```python
from build123d import *

# Parameters (mm, degrees)
F0_W     = 3.5
F0_H     = 11
F1_DEPTH = 10
F2_R     = 3
F3_R     = 15.5
F4_DEPTH = 25
F3_W     = 3.5
F3_H     = 5
F5_DEPTH = 3
F6_R     = 2
F7_R     = 15.5
F8_DEPTH = 10


with BuildPart() as f1:
    # F0 (on Top) → F1 (new body)
    with BuildSketch(Plane.XY):
        with BuildLine():
            ThreePointArc((0, -19.5), (13.7885822331, -13.7885822331), (19.5, 0))
            ThreePointArc((19.5, 0), (13.7885822331, 13.7885822331), (0, 19.5))
            ThreePointArc((0, 19.5), (-19.5, 0), (0, -19.5))
        make_face()
        with BuildLine():
            ThreePointArc((0, 19.5), (13.7885822331, 13.7885822331), (19.5, 0))
            ThreePointArc((19.5, 0), (13.7885822331, -13.7885822331), (0, -19.5))
            Line((0, -19.5), (21.5, -19.5))
            Line((21.5, -19.5), (21.5, 19.5))
            Line((21.5, 19.5), (0, 19.5))
        make_face()
        Polygon((30.5, 16), (21.5, 19.5), (21.5, -19.5), (30.5, -16), (30.5, -5.5), (30.5, 5.5), align=None)
        with Locations((32.25, 0)):
            Rectangle(F0_W, F0_H)
    extrude(amount=F1_DEPTH)

    # F2
    f2_edges = [f1.edges().sort_by_distance(p)[0] for p in [
        (30.5, 16, 5),
        (21.5, 19.5, 5),
        (30.5, -16, 5),
        (21.5, -19.5, 5),
    ]]
    fillet(f2_edges, radius=F2_R)

    # F3 (on face) → F4 (cut)
    with BuildSketch(Plane.XY.offset(10)):
        Circle(F3_R)
        with BuildLine():
            Line((20.9371966075, 16.5), (10.3923048454, 16.5))
            ThreePointArc((10.3923048454, 16.5), (17.0719059347, 9.4233766643), (19.5, 0))
            ThreePointArc((19.5, 0), (17.0719059347, -9.4233766643), (10.3923048454, -16.5))
            Line((10.3923048454, -16.5), (20.9371966075, -16.5))
            Line((20.9371966075, -16.5), (27.5, -13.9477986807))
            Line((27.5, -13.9477986807), (27.5, -2.5))
            Line((27.5, -2.5), (27.5, 2.5))
            Line((27.5, 2.5), (27.5, 13.9477986807))
            Line((27.5, 13.9477986807), (20.9371966075, 16.5))
        make_face()
    extrude(amount=-F4_DEPTH, mode=Mode.SUBTRACT)

    # F3 (on face) → F5 (join)
    with BuildSketch(Plane.XY.offset(10)):
        with BuildLine():
            Line((20.9371966075, 24.5), (0, 24.5))
            ThreePointArc((0, 24.5), (-24.5, 0), (0, -24.5))
            Line((0, -24.5), (20.9371966075, -24.5))
            ThreePointArc((20.9371966075, -24.5), (22.4122730498, -24.3628334263), (23.8367666967, -23.9560373723))
            Line((23.8367666967, -23.9560373723), (30.3995700892, -21.403836053))
            ThreePointArc((30.3995700892, -21.403836053), (34.1028993902, -18.4646249606), (35.5, -13.9477986807))
            Line((35.5, -13.9477986807), (35.5, -10.5))
            Line((35.5, -10.5), (39, -10.5))
            Line((39, -10.5), (39, 10.5))
            Line((39, 10.5), (35.5, 10.5))
            Line((35.5, 10.5), (35.5, 13.9477986807))
            ThreePointArc((35.5, 13.9477986807), (34.1028993902, 18.4646249606), (30.3995700892, 21.403836053))
            Line((30.3995700892, 21.403836053), (23.8367666967, 23.9560373723))
            ThreePointArc((23.8367666967, 23.9560373723), (22.4122730498, 24.3628334263), (20.9371966075, 24.5))
        make_face()
        with BuildLine():
            ThreePointArc((0, -19.5), (-19.5, 0), (0, 19.5))
            Line((0, 19.5), (20.9371966075, 19.5))
            ThreePointArc((20.9371966075, 19.5), (21.4903502734, 19.4485625349), (22.024535391, 19.2960140146))
            Line((22.024535391, 19.2960140146), (28.5873387835, 16.7438126953))
            ThreePointArc((28.5873387835, 16.7438126953), (29.9760872713, 15.6416085357), (30.5, 13.9477986807))
            Line((30.5, 13.9477986807), (30.5, 5.5))
            Line((30.5, 5.5), (34, 5.5))
            Line((34, 5.5), (34, -5.5))
            Line((34, -5.5), (30.5, -5.5))
            Line((30.5, -5.5), (30.5, -13.9477986807))
            ThreePointArc((30.5, -13.9477986807), (29.9760872713, -15.6416085357), (28.5873387835, -16.7438126953))
            Line((28.5873387835, -16.7438126953), (22.024535391, -19.2960140146))
            ThreePointArc((22.024535391, -19.2960140146), (21.4903502734, -19.4485625349), (20.9371966075, -19.5))
            Line((20.9371966075, -19.5), (0, -19.5))
        make_face(mode=Mode.SUBTRACT)
        with BuildLine():
            ThreePointArc((0, -16.5), (-16.5, 0), (0, 16.5))
            Line((0, 16.5), (10.3923048454, 16.5))
            ThreePointArc((10.3923048454, 16.5), (5.4083269132, 18.7349939952), (0, 19.5))
            ThreePointArc((0, 19.5), (-19.5, 0), (0, -19.5))
            ThreePointArc((0, -19.5), (5.4083269132, -18.7349939952), (10.3923048454, -16.5))
            Line((10.3923048454, -16.5), (0, -16.5))
        make_face()
        with Locations((29.25, 0)):
            Rectangle(F3_W, F3_H)
        with BuildLine():
            ThreePointArc((0, 19.5), (5.4083269132, 18.7349939952), (10.3923048454, 16.5))
            Line((10.3923048454, 16.5), (20.9371966075, 16.5))
            Line((20.9371966075, 16.5), (27.5, 13.9477986807))
            Line((27.5, 13.9477986807), (27.5, 2.5))
            Line((27.5, 2.5), (31, 2.5))
            Line((31, 2.5), (31, -2.5))
            Line((31, -2.5), (27.5, -2.5))
            Line((27.5, -2.5), (27.5, -13.9477986807))
            Line((27.5, -13.9477986807), (20.9371966075, -16.5))
            Line((20.9371966075, -16.5), (10.3923048454, -16.5))
            ThreePointArc((10.3923048454, -16.5), (5.4083269132, -18.7349939952), (0, -19.5))
            Line((0, -19.5), (20.9371966075, -19.5))
            ThreePointArc((20.9371966075, -19.5), (21.4903502734, -19.4485625349), (22.024535391, -19.2960140146))
            Line((22.024535391, -19.2960140146), (28.5873387835, -16.7438126953))
            ThreePointArc((28.5873387835, -16.7438126953), (29.9760872713, -15.6416085357), (30.5, -13.9477986807))
            Line((30.5, -13.9477986807), (30.5, -5.5))
            Line((30.5, -5.5), (34, -5.5))
            Line((34, -5.5), (34, 5.5))
            Line((34, 5.5), (30.5, 5.5))
            Line((30.5, 5.5), (30.5, 13.9477986807))
            ThreePointArc((30.5, 13.9477986807), (29.9760872713, 15.6416085357), (28.5873387835, 16.7438126953))
            Line((28.5873387835, 16.7438126953), (22.024535391, 19.2960140146))
            ThreePointArc((22.024535391, 19.2960140146), (21.4903502734, 19.4485625349), (20.9371966075, 19.5))
            Line((20.9371966075, 19.5), (0, 19.5))
        make_face()
        with BuildLine():
            Line((20.9371966075, 16.5), (10.3923048454, 16.5))
            ThreePointArc((10.3923048454, 16.5), (17.0719059347, 9.4233766643), (19.5, 0))
            ThreePointArc((19.5, 0), (17.0719059347, -9.4233766643), (10.3923048454, -16.5))
            Line((10.3923048454, -16.5), (20.9371966075, -16.5))
            Line((20.9371966075, -16.5), (27.5, -13.9477986807))
            Line((27.5, -13.9477986807), (27.5, -2.5))
            Line((27.5, -2.5), (27.5, 2.5))
            Line((27.5, 2.5), (27.5, 13.9477986807))
            Line((27.5, 13.9477986807), (20.9371966075, 16.5))
        make_face()
        with BuildLine():
            Line((10.3923048454, 16.5), (0, 16.5))
            ThreePointArc((0, 16.5), (11.6672618896, 11.6672618896), (16.5, 0))
            ThreePointArc((16.5, 0), (11.6672618896, -11.6672618896), (0, -16.5))
            Line((0, -16.5), (10.3923048454, -16.5))
            ThreePointArc((10.3923048454, -16.5), (17.0719059347, -9.4233766643), (19.5, 0))
            ThreePointArc((19.5, 0), (17.0719059347, 9.4233766643), (10.3923048454, 16.5))
        make_face()
        with BuildLine():
            ThreePointArc((16.5, 0), (11.6672618896, 11.6672618896), (0, 16.5))
            ThreePointArc((0, 16.5), (-16.5, 0), (0, -16.5))
            ThreePointArc((0, -16.5), (11.6672618896, -11.6672618896), (16.5, 0))
        make_face()
        Circle(F3_R, mode=Mode.SUBTRACT)
    extrude(amount=F5_DEPTH)

    # F6
    f6_edges = [f1.edges().sort_by_distance(p)[0] for p in [
        (-19.5, 0, 0),
        (10.468598, -19.5, 0),
        (25.305937, -18.019913, 0),
        (30.5, -9.723899, 0),
        (29.976087, -15.641609, 0),
        (34, 0, 0),
        (32.25, 5.5, 0),
        (30.5, 9.723899, 0),
        (21.49035, -19.448563, 0),
        (10.468598, 19.5, 0),
        (25.305937, 18.019913, 0),
        (29.976087, 15.641609, 0),
        (21.49035, 19.448563, 0),
        (32.25, -5.5, 0),
    ]]
    fillet(f6_edges, radius=F6_R)

    # F7 (on face) → F8 (join)
    with BuildSketch(Plane(origin=(0, 0, 0), x_dir=(1, 0, 0), z_dir=(0, 0, -1))):
        with BuildLine():
            ThreePointArc((0, -17.5), (12.3743686708, -12.3743686708), (17.5, 0))
            ThreePointArc((17.5, 0), (12.3743686708, 12.3743686708), (0, 17.5))
            ThreePointArc((0, 17.5), (-17.5, 0), (0, -17.5))
        make_face()
        Circle(F7_R, mode=Mode.SUBTRACT)
    extrude(amount=F8_DEPTH)


solid = f1.part
```
The listing builds one solid part. Answer for the finished solid, in the listing's coordinates (mm). A direction names the side the tool comes from. Coordinates: 2 decimals unless noted, no trailing zeros. Loops run counter-clockwise (first coordinate to the right, second up) from the corner with the lowest first, then second, coordinate; pieces in that order, holes last. Notation, with made-up numbers: M -39.5,-38 L -8.5,-38 A19 ccw -8.5,-10 Z; hole C -30.75,-35 d3. An arc over 180 degrees is marked long. Answer as CSV lines item,"result". Start each with the question number.
(1) Given pin 1 (8 mm diameter, centred on x = -12.5, z = -0.5, fed in from +Y); pin 2 (2.5 mm diameter, centred on y = -8, z = 7.5, fed in from +X); pin 3 (0.9 mm diameter, centred on y = -13, z = 12, fed in from +X), each flat-ended and moving along its own axis, determine where each tip first touches the part or whether it passes through.
(2) Find the intervals of material crossed by L1, parallel to X at y = 11.5, z = 6.25; L2, parallel to X at y = 1.5, z = 9.5; L3, parallel to Y at x = 0, z = -1.25, in increasing order. Write a range as [from, to].
(3) For faces 1 (the flat face through (21, 0, 10)), 2 (the flat face through (19, 0, 0)), 3 (the cylindrical face through (29.962, -15.662, 6.056)), 4 (the flat face through (35.5, 12, 11)), determine the directions among +Z, -Z, +X, -X, +Y, -Y from which every point of the face is accessible in a straight line to the end or side of a thin tool.
(4) The part is cut by section C-C (z = -4.25). Give the vertices of the cut face in (x, y), and give its area (3 significant figures).
(5) The part is cut by section D-D (x = 12). Give the vertices of the cut face in (y, z), and give its area (3 significant figures).
(6) The part is cut by section B-B (z = 7). Give the vertices of the cut face in (x, y).
(7) The mould has two halves that part along Y. Classify faces 5 (the cylindrical face through (-2.018, -15.368, 1.661)), 6 (the cylindrical face through (22.43, 24.36, 11.48)), 7 (the cylindrical face through (34.065, -18.52, 11.479)): pulls with the +Y half, pulls with the -Y half, needs draft (parallel to the pull), parting line crosses it, or undercut.
(8) The part is cut by section A-A (x = 5). Give the vertices of the cut face in (y, z).
Determined:
1,pin 1,"y = 17.21"
1,pin 2,"x = 30.5"
1,pin 3,"x = 35.5"
2,L1,"[-15.75, -10.39], [10.39, 15.75], [27.5, 30.5]"
2,L2,"[-19.44, -15.43], [15.43, 19.44], [27.5, 34]"
2,L3,"[-17.5, -15.5], [15.5, 17.5]"
3,face 1,"-Z"
3,face 2,"-Z, +X"
3,face 3,"-Z, +X, -Y"
3,face 4,"+Z, -Z, +X, +Y"
4,outline,"C 0,0 d35; hole C 0,0 d31"
4,area,"207 mm2"
5,outline,"M -24.5,10 L -19.5,10 L -19.5,2 A2 ccw -17.5,0 L -16.5,0 L -16.5,10 L -15.37,10 L -15.37,0 L -12.74,0 L -12.74,-10 L -9.81,-10 L -9.81,13 L -24.5,13 Z; M 9.81,-10 L 12.74,-10 L 12.74,0 L 15.37,0 L 15.37,10 L 16.5,10 L 16.5,0 L 17.5,0 A2 ccw 19.5,2 L 19.5,10 L 24.5,10 L 24.5,13 L 9.81,13 Z"
5,area,"316 mm2"
6,outline,"M 0,-19.5 L 20.94,-19.5 A3 ccw 22.02,-19.3 L 28.59,-16.74 A3 ccw 30.5,-13.95 L 30.5,-5.5 L 34,-5.5 L 34,5.5 L 30.5,5.5 L 30.5,13.95 A3 ccw 28.59,16.74 L 22.02,19.3 A3 ccw 20.94,19.5 L 0,19.5 A19.5 ccw Z; hole C 0,0 d31; hole M 10.39,-16.5 L 20.94,-16.5 L 27.5,-13.95 L 27.5,13.95 L 20.94,16.5 L 10.39,16.5 A19.5 cw Z"
7,face 5,"undercut"
7,face 6,"pulls with the +Y half"
7,face 7,"pulls with the -Y half"
8,outline,"M -24.5,10 L -19.5,10 L -19.5,2 A2 ccw -17.5,0 L -16.77,0 L -16.77,-10 L -14.67,-10 L -14.67,13 L -24.5,13 Z; M 14.67,-10 L 16.77,-10 L 16.77,0 L 17.5,0 A2 ccw 19.5,2 L 19.5,10 L 24.5,10 L 24.5,13 L 14.67,13 Z"
